```python
from build123d import *

# Parameters (mm, degrees)
F0_R          = 7
F1_DEPTH      = 1
F3_DEPTH      = 10.5
F4_R          = 7
F5_DEPTH      = 1
F6_R          = 2.5
F7_DEPTH      = 5
F7_DEPTH_BACK = 17.5


with BuildPart() as f1:
    # F0 (on Top) → F1 (new body)
    with BuildSketch(Plane.XY):
        Circle(F0_R)
    extrude(amount=F1_DEPTH)

    # F2 (on face) → F3 (join)
    with BuildSketch(Plane.XY.offset(1)):
        with BuildLine():
            ThreePointArc((0.829134, 4.168337), (0.416573, 4.229535), (0, 4.25))
            Line((0, 4.25), (0, 5))
            ThreePointArc((0, 5), (-0.490086, 4.975924), (-0.975452, 4.903926))
            Line((-0.975452, 4.903926), (-0.829134, 4.168337))
            ThreePointArc((-0.829134, 4.168337), (-1.23371, 4.066996), (-1.626405, 3.926488))
            Line((-1.626405, 3.926488), (-1.913417, 4.619398))
            ThreePointArc((-1.913417, 4.619398), (-2.356984, 4.409606), (-2.777851, 4.157348))
            Line((-2.777851, 4.157348), (-2.361173, 3.533746))
            ThreePointArc((-2.361173, 3.533746), (-2.696171, 3.285294), (-3.005204, 3.005204))
            Line((-3.005204, 3.005204), (-3.535534, 3.535534))
            ThreePointArc((-3.535534, 3.535534), (-3.865052, 3.171966), (-4.157348, 2.777851))
            Line((-4.157348, 2.777851), (-3.533746, 2.361173))
            ThreePointArc((-3.533746, 2.361173), (-3.748165, 2.003436), (-3.926488, 1.626405))
            Line((-3.926488, 1.626405), (-4.619398, 1.913417))
            ThreePointArc((-4.619398, 1.913417), (-4.784702, 1.451423), (-4.903926, 0.975452))
            Line((-4.903926, 0.975452), (-4.168337, 0.829134))
            ThreePointArc((-4.168337, 0.829134), (-4.229535, 0.416573), (-4.25, 0))
            Line((-4.25, 0), (-5, 0))
            ThreePointArc((-5, 0), (-4.975924, -0.490086), (-4.903926, -0.975452))
            Line((-4.903926, -0.975452), (-4.168337, -0.829134))
            ThreePointArc((-4.168337, -0.829134), (-4.066996, -1.23371), (-3.926488, -1.626405))
            Line((-3.926488, -1.626405), (-4.619398, -1.913417))
            ThreePointArc((-4.619398, -1.913417), (-4.409606, -2.356984), (-4.157348, -2.777851))
            Line((-4.157348, -2.777851), (-3.533746, -2.361173))
            ThreePointArc((-3.533746, -2.361173), (-3.285294, -2.696171), (-3.005204, -3.005204))
            Line((-3.005204, -3.005204), (-3.535534, -3.535534))
            ThreePointArc((-3.535534, -3.535534), (-3.171966, -3.865052), (-2.777851, -4.157348))
            Line((-2.777851, -4.157348), (-2.361173, -3.533746))
            ThreePointArc((-2.361173, -3.533746), (-2.003436, -3.748165), (-1.626405, -3.926488))
            Line((-1.626405, -3.926488), (-1.913417, -4.619398))
            ThreePointArc((-1.913417, -4.619398), (-1.451423, -4.784702), (-0.975452, -4.903926))
            Line((-0.975452, -4.903926), (-0.829134, -4.168337))
            ThreePointArc((-0.829134, -4.168337), (-0.416573, -4.229535), (0, -4.25))
            Line((0, -4.25), (0, -5))
            ThreePointArc((0, -5), (0.490086, -4.975924), (0.975452, -4.903926))
            Line((0.975452, -4.903926), (0.829134, -4.168337))
            ThreePointArc((0.829134, -4.168337), (1.23371, -4.066996), (1.626405, -3.926488))
            Line((1.626405, -3.926488), (1.913417, -4.619398))
            ThreePointArc((1.913417, -4.619398), (2.356984, -4.409606), (2.777851, -4.157348))
            Line((2.777851, -4.157348), (2.361173, -3.533746))
            ThreePointArc((2.361173, -3.533746), (2.696171, -3.285294), (3.005204, -3.005204))
            Line((3.005204, -3.005204), (3.535534, -3.535534))
            ThreePointArc((3.535534, -3.535534), (3.865052, -3.171966), (4.157348, -2.777851))
            Line((4.157348, -2.777851), (3.533746, -2.361173))
            ThreePointArc((3.533746, -2.361173), (3.748165, -2.003436), (3.926488, -1.626405))
            Line((3.926488, -1.626405), (4.619398, -1.913417))
            ThreePointArc((4.619398, -1.913417), (4.784702, -1.451423), (4.903926, -0.975452))
            Line((4.903926, -0.975452), (4.168337, -0.829134))
            ThreePointArc((4.168337, -0.829134), (4.229535, -0.416573), (4.25, 0))
            Line((4.25, 0), (5, 0))
            ThreePointArc((5, 0), (4.975924, 0.490086), (4.903926, 0.975452))
            Line((4.903926, 0.975452), (4.168337, 0.829134))
            ThreePointArc((4.168337, 0.829134), (4.066996, 1.23371), (3.926488, 1.626405))
            Line((3.926488, 1.626405), (4.619398, 1.913417))
            ThreePointArc((4.619398, 1.913417), (4.409606, 2.356984), (4.157348, 2.777851))
            Line((4.157348, 2.777851), (3.533746, 2.361173))
            ThreePointArc((3.533746, 2.361173), (3.285294, 2.696171), (3.005204, 3.005204))
            Line((3.005204, 3.005204), (3.535534, 3.535534))
            ThreePointArc((3.535534, 3.535534), (3.171966, 3.865052), (2.777851, 4.157348))
            Line((2.777851, 4.157348), (2.361173, 3.533746))
            ThreePointArc((2.361173, 3.533746), (2.003436, 3.748165), (1.626405, 3.926488))
            Line((1.626405, 3.926488), (1.913417, 4.619398))
            ThreePointArc((1.913417, 4.619398), (1.451423, 4.784702), (0.975452, 4.903926))
            Line((0.975452, 4.903926), (0.829134, 4.168337))
        make_face()
    extrude(amount=F3_DEPTH)

    # F4 (on face) → F5 (join)
    with BuildSketch(Plane.XY.offset(11.5)):
        with Locations((0, 0.452107)):
            Circle(F4_R)
    extrude(amount=F5_DEPTH)

    # F6 (on face) → F7 (join, two sides)
    with BuildSketch(Plane(origin=(0, 0, 0), x_dir=(1, 0, 0), z_dir=(0, 0, -1))) as f7_sk:
        Circle(F6_R)
    extrude(amount=F7_DEPTH)
    extrude(f7_sk.sketch, amount=-F7_DEPTH_BACK)


solid = f1.part
```
Read the model definition and answer for the solid it produces. Units are mm, in the model's axes. A direction names the side the tool comes from. Coordinates: 2 decimals unless noted, no trailing zeros. Write each loop counter-clockwise with the first axis right and the second up, starting at its lowest first coordinate (ties: lowest second). Pieces come first, ordered by that corner, then holes. Notation, with made-up numbers: (-19.5, 45.25) -> (-6.5, 45.25) arc R13 ccw to (-6.5, 65.25) -> close; hole circle Ø4 at (-38, -24). An arc over 180 degrees is marked (long way). Return JSON: item names as keys, results as strings.
1. Determine the mould class of faces 6 (the face through (-0.54, 2.44, 14.96)), 7 (the face through (-4.783, 1.458, 6.176)), 8 (the face through (0, -3, 0)) for opening direction Z: pulls with the +Z half, pulls with the -Z half, needs draft (parallel to the pull), parting line crosses it, or undercut.
Found:
{"face 6": "needs draft", "face 7": "undercut", "face 8": "pulls with the -Z half"}
2. A cutting plane is placed at A-A (y = 3.25). Determine the outline of the cut face in (x, z), and give its area (3 significant figures).
Found:
{"outline": "(-6.42, 11.5) -> (-3.8, 11.5) -> (-3.8, 1) -> (-6.2, 1) -> (-6.2, 0) -> (6.2, 0) -> (6.2, 1) -> (3.25, 1) -> (3.25, 11.5) -> (6.42, 11.5) -> (6.42, 12.5) -> (-6.42, 12.5) -> close; hole (-3.25, 1) -> (-2.74, 1) -> (-2.74, 11.5) -> (-3.25, 11.5) -> close", "area": "93.9 mm2"}
3. A tool of negligible diameter and unlimited length cuts with its end or side. For faces 1 (the face through (-1.52, -6.38, 11.99)), 2 (the face through (4.23, -0.42, 6.18)), 3 (the face through (-4.977, -0.483, 6.176)), 4 (the face through (1.458, 4.783, 6.176)), 5 (the face through (6.466, -2.681, 0.493)), from which of +Z, -Z, +X, -X, +Y, -Y can it reach the whole face along a straight path? Write none if from no direction.
Found:
{"face 1": "+Z", "face 2": "+X", "face 3": "-X, -Y", "face 4": "+X, +Y", "face 5": "-Z"}
4. Each of these flat-tipped pins is pushed along its axis until it touches: P1, Ø1, axis at x = 3.5, z = 8, coming from the +Y side; P2, Ø4, axis at x = -4, y = 1, coming from the -Z side; P3, Ø1.5, axis at y = 0, z = 2, coming from the +X side; P4, Ø3, axis at x = -1, z = 13, coming from the -Y side. Where does it stop, or does it pass through?
Found:
{"P1": "y = 4", "P2": "z = -5", "P3": "x = 5", "P4": "y = -6.55"}
5. Find the intervals of material crossed by line 1 along Z through (x, y) = (-1.25, -5.25); line 2 along Z through (x, y) = (1.75, 2.25); line 3 along Y through (x, z) = (3.75, 3.75), in increasing order. Write a range as from..to.
Found:
{"line 1": "0..1, 11.5..12.5", "line 2": "0..12.5", "line 3": "-3.31..-2.51, -2..2.51"}
6. A cutting plane is placed at B-B (y = -1.25). Determine the outline of the cut face in (x, z), and give its area (3 significant figures).
Found:
{"outline": "(-6.89, 0) -> (-2.17, 0) -> (-2.17, -5) -> (2.17, -5) -> (2.17, 0) -> (6.89, 0) -> (6.89, 1) -> (4.84, 1) -> (4.84, 11.5) -> (6.79, 11.5) -> (6.79, 12.5) -> (2.17, 12.5) -> (2.17, 17.5) -> (-2.17, 17.5) -> (-2.17, 12.5) -> (-6.79, 12.5) -> (-6.79, 11.5) -> (-4.06, 11.5) -> (-4.06, 1) -> (-6.89, 1) -> close", "area": "164 mm2"}
